Part model, mm, in its own coordinate system. Face numbers are marked on the shaded views. A direction names the side the tool comes from. Give positions to 0.01 mm unless a question says otherwise; leave off trailing zeros. Write each loop counter-clockwise with the first axis right and the second up, starting at its lowest first coordinate (ties: lowest second). Pieces come first, ordered by that corner, then holes.
from build123d import *

# Parameters (mm, degrees)
SKETCH3_W = 3.4
SKETCH3_H = 25


with BuildPart() as part:
    # Sketch1 → Revolve1 (revolve)
    with BuildSketch(Plane.XY):
        Polygon((-6, 23.256587884), (-6, 6.256587884), (-5.8, 6.056587884), (0, 6.056587884), (0, 31.056587884), (-8, 31.056587884), (-8, 24.756587884), (-6.5, 23.256587884), align=None)
    revolve(axis=Axis((0, 31.056587884, 0), (0, -1, 0)))

    # Sketch3 → M8x1.25 Tapped Hole1 (revolve, cut)
    with BuildSketch(Plane(origin=(0, 31.056587884, 0), x_dir=(0, 0, 1), z_dir=(1, 0, 0))):
        with Locations((1.7, 12.5)):
            Rectangle(SKETCH3_W, SKETCH3_H)
    revolve(axis=Axis((0, 37.406587884, 0), (0, -1, 0)), mode=Mode.SUBTRACT)


solid = part.part
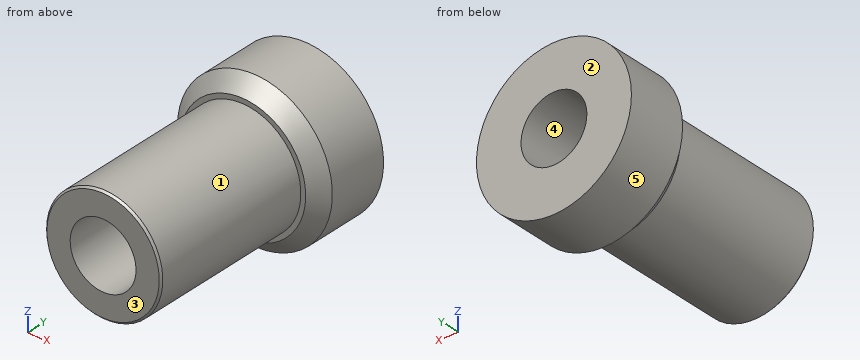
1) Mould opens along Z. For the marked faces 3, 4 and 5 say: +Z half, -Z half, draft (parallel to the pull), parting line (faces both ways), or undercut.
Check result:
face 3: draft
face 4: undercut
face 5: parting line
2) Saw through at B-B (x = 0). Write the cut outline in (y, z), and give its area (3 significant figures).
Check result:
outline: (6.06, -5.8) - (6.26, -6) - (23.26, -6) - (23.26, -6.5) - (24.76, -8) - (31.06, -8) - (31.06, -3.4) - (6.06, -3.4) - close; (6.06, 3.4) - (31.06, 3.4) - (31.06, 8) - (24.76, 8) - (23.26, 6.5) - (23.26, 6) - (6.26, 6) - (6.06, 5.8) - close
area: 159 mm2
3) Saw through at A-A (z = 0). Write the cut outline in (x, y), and give its area (3 significant figures).
Check result:
outline: (-8, 24.76) - (-6.5, 23.26) - (-6, 23.26) - (-6, 6.26) - (-5.8, 6.06) - (-3.4, 6.06) - (-3.4, 31.06) - (-8, 31.06) - close; (3.4, 6.06) - (5.8, 6.06) - (6, 6.26) - (6, 23.26) - (6.5, 23.26) - (8, 24.76) - (8, 31.06) - (3.4, 31.06) - close
area: 159 mm2
4) Saw through at C-C (y = 10.5). Write the cut outline in (x, z), and give its area (3 significant figures).
Check result:
outline: circle Ø12 at (0, 0); hole circle Ø6.8 at (0, 0)
area: 76.8 mm2
5) 3-axis set-ups, long thin cutter, end or side, ignore diameter. For the marked faces 1 and 2: which of +Z, -Z, +X, -X, +Y, -Y reach the whole face in a straight line?
Check result:
face 1: -Y
face 2: +Z, -Z, +X, -X, +Y
6) Flat gauge pins, fed straight in: P1, Ø5, axis at y = 26.5, z = -4, coming from the -X side; P2, Ø6, axis at x = -4.5, y = 23, coming from the -Z side; P3, Ø8, axis at y = 15, z = -5, coming from the -X side. Where does each tip first touch, or does it go through?
Check result:
P1: stops at x = -7.86
P2: stops at z = -7.73
P3: stops at x = -5.92
7) Drill centre lines: L1, parallel to Z at x = 0, y = 15.25; L2, parallel to X at y = 20.5, z = 2. Where is each one in solid material? Low to high.
Check result:
L1: z = -6 to -3.4, 3.4 to 6
L2: x = -5.66 to -2.75, 2.75 to 5.66
